from build123d import *

# Parameters (mm, degrees)
F0_R      = 4.15
F1_DEPTH  = 60
F0_R_2    = 7
F1_FACE_R = 4.15
F2_DEPTH  = 5
F4_D      = 5
F4_DEPTH  = 15
F4_TIP    = 1.5021515476


with BuildPart() as f1:
    # F0 (on Front) → F1 (new body)
    with BuildSketch(Plane.XZ):
        Circle(F0_R)
    extrude(amount=F1_DEPTH)

    # F0 (on Front) + F1_face (on face) → F2 (join)
    with BuildSketch(Plane.XZ):
        Circle(F0_R_2)
        Circle(F0_R, mode=Mode.SUBTRACT)
    with BuildSketch(Plane(origin=(0, 0, 0), x_dir=(1, 0, 0), z_dir=(0, 1, 0))):
        Circle(F1_FACE_R)
    extrude(amount=-F2_DEPTH, dir=(0, -1, 0))

    # F4
    with Locations(Plane.XZ.offset(60)):
        with Locations((0, 0)):
            Hole(F4_D / 2, depth=F4_DEPTH)
            with Locations((0, 0, -(F4_DEPTH + F4_TIP / 2))):  # 118° drill point
                Cone(0, F4_D / 2, F4_TIP, mode=Mode.SUBTRACT)


solid = f1.part
Geometry check sheet. Reference: the model listing, model coordinates, mm. A direction names the side the tool comes from. Give positions to 0.01 mm unless a question says otherwise; leave off trailing zeros. Loops run counter-clockwise (first coordinate to the right, second up) from the corner with the lowest first, then second, coordinate; pieces in that order, holes last.
(1) Section check A-A on y = -54.5. Record the cut outline in (x, z), then the cut area to 3 significant figures.
From the geometry:
outline: circle Ø8.3 at (0, 0); hole circle Ø5 at (0, 0)
area: 34.5 mm2
(2) Release check for a two-part mould opening along X. For faces 1 (the cylindrical face through (-0.9, -29.58, -4.05)), 2 (the flat face through (0, 0, -5)), 3 (the conical face through (-0.094, -43.759, -0.424)) record: released by +X, released by -X, zero draft, split by the parting line, or undercut.
From the geometry:
face 1: split by the parting line
face 2: zero draft
face 3: undercut
(3) Section check D-D on y = -8. Record the cut outline in (x, z).
From the geometry:
outline: circle Ø8.3 at (0, 0)
(4) Set-up check for faces 4 (the cylindrical face through (6.466, 2.465, -2.681)), 5 (the cylindrical face through (0.54, -52.4, -2.44)): record each of +Z, -Z, +X, -X, +Y, -Y from which the full face is reachable in a straight line by a thin tool's end or side.
From the geometry:
face 4: +Y, -Y
face 5: -Y
(5) Section check B-B on x = -5.5. Record the cut outline in (y, z), then the cut area to 3 significant figures.
From the geometry:
outline: (0, -4.33) - (5, -4.33) - (5, 4.33) - (0, 4.33) - close
area: 43.3 mm2
(6) Depth check by flat-ended pin: pin 1 Ø1.5 at (x, y) = (-3, -3.5) entering from -Z; pin 2 Ø3 at (x, y) = (0, -38) entering from +Z; pin 3 Ø3 at (y, z) = (-5, 1.5) entering from -X. Enter the tip coordinate at first touch or a pass-through.
From the geometry:
pin 1: stops at z = -3.49
pin 2: stops at z = 4.15
pin 3: stops at x = -4.15
(7) Thickness scan on L1, parallel to Z at x = 0, y = -57; L2, parallel to Y at x = -4.25, z = -1.25; L3, parallel to Z at x = -0.25, y = -27. Record the ranges inside material, lowest first.
From the geometry:
L1: z = -4.15 to -2.5, 2.5 to 4.15
L2: y = 0 to 5
L3: z = -4.14 to 4.14
(8) Section check C-C on z = 5. Record the cut outline in (x, y), then the cut area to 3 significant figures.
From the geometry:
outline: (-4.9, 0) - (4.9, 0) - (4.9, 5) - (-4.9, 5) - close
area: 49.0 mm2
